Can you work these out from the drawing? Everything is in mm from the part's minimum corner. A direction names the side the tool comes from. Round coordinates to 2 decimals unless told otherwise and drop trailing zeros. Write each loop counter-clockwise with the first axis right and the second up, starting at its lowest first coordinate (ties: lowest second). Pieces come first, ordered by that corner, then holes. Notation, with made-up numbers: M 72.5,17 L 116.5,17 A31 ccw 116.5,47 Z; hole C 2,-34.75 d8. An arc over 180 degrees is marked long. Use one line per item in the form item = value. Start each with the question number.
Q1. I want a section at C-C on z = 22.5. List the corners of the cut face in (x, y) for me.
Q2. I need wall thicknesses on line 1 along X through (y, z) = (17.5, 11); line 2 along Y through (x, z) = (25, 23); line 3 along X through (y, z) = (80, 29). Which ranges of each line are inside material? Lowest first, please. Write a range as from..to.
Q3. I'm going to push flat-ended pins straight in: pin 1 Ø11.5 at (y, z) = (27.5, 15) entering from +X; pin 2 Ø1.5 at (x, y) = (37, 2) entering from -Z; pin 3 Ø6 at (x, y) = (31.5, 30.5) entering from -Z. Where does each tip first touch, or does it pass through?
Q4. We'd pull the mould along Y, two halves only. Please class the marked faces 3, 4 and 5: +Y half, -Y half, draft (parallel to the pull), parting line (faces both ways), or undercut.
Q5. I want a section at D-D on y = 80.5. List the corners of the cut face in (x, z) for me.
Q6. For the marked faces 1 and 2, which set-ups out of +Z, -Z, +X, -X, +Y, -Y let a thin tool reach every point of the face, with its end or its side?
Q7. I want a section at B-B on x = 39.5. List the corners of the cut face in (y, z) for me.
Q8. I want a section at A-A on y = 36.5. List the corners of the cut face in (x, z) for me.
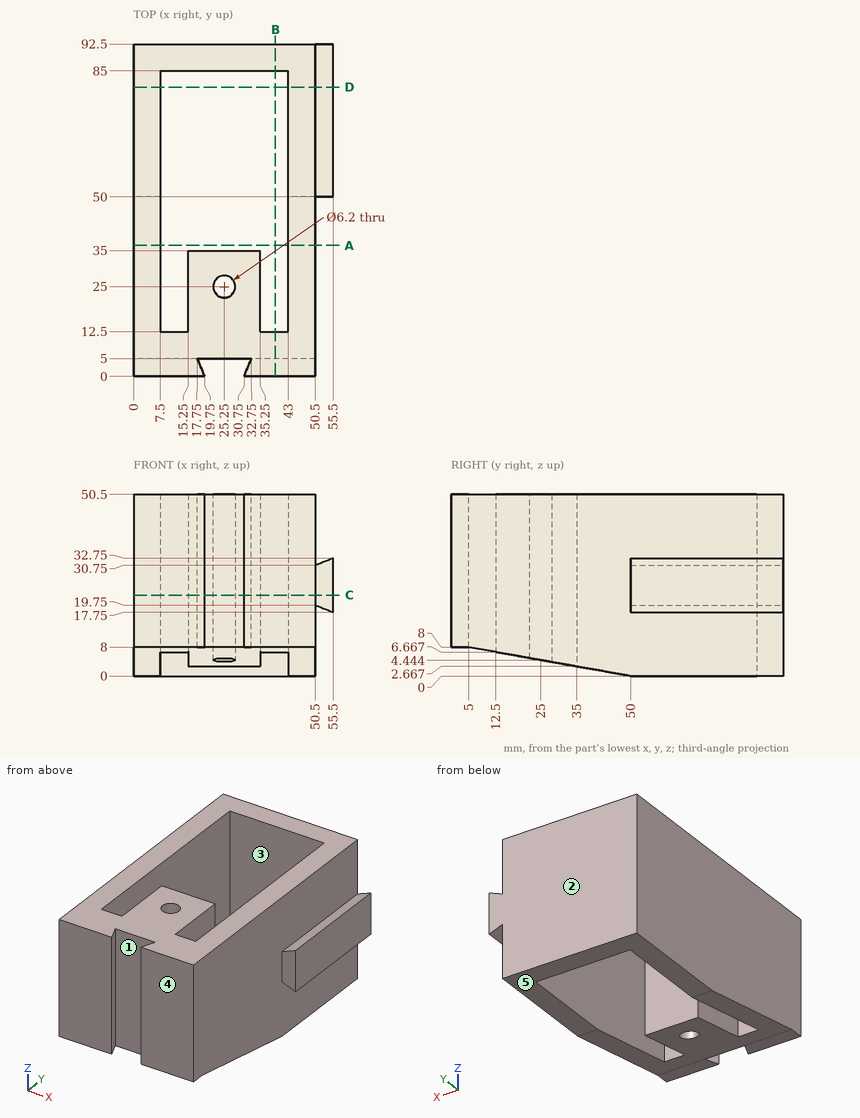
Reported:
q1.outline = M 0,0 L 19.75,0 L 17.75,5 L 32.75,5 L 30.75,0 L 50.5,0 L 50.5,50 L 55.5,50 L 55.5,92.5 L 0,92.5 Z; hole M 7.5,12.5 L 15.25,12.5 L 15.25,35 L 35.25,35 L 35.25,12.5 L 43,12.5 L 43,85 L 7.5,85 Z; hole C 25.25,25 d6.2
q2.line_1 = 0..7.5, 15.25..35.25, 43..50.5
q2.line_2 = 5..21.91, 28.09..35, 85..92.5
q2.line_3 = 0..7.5, 43..55.5
q3.pin_1 = 50.5
q3.pin_2 = 8
q3.pin_3 = 2.93
q4.face_3 = undercut
q4.face_4 = -Y half
q4.face_5 = draft
q5.outline = M 0,0 L 7.5,0 L 7.5,50.5 L 0,50.5 Z; M 43,0 L 50.5,0 L 50.5,19.75 L 55.5,17.75 L 55.5,32.75 L 50.5,30.75 L 50.5,50.5 L 43,50.5 Z
q6.face_1 = +Z, -Z
q6.face_2 = +Z, -Z, +X, -X, +Y
q7.outline = M 0,8 L 5,8 L 12.5,6.67 L 12.5,50.5 L 0,50.5 Z; M 85,0 L 92.5,0 L 92.5,50.5 L 85,50.5 Z
q8.outline = M 0,2.4 L 7.5,2.4 L 7.5,50.5 L 0,50.5 Z; M 43,2.4 L 50.5,2.4 L 50.5,50.5 L 43,50.5 Z
